Verification items for the finished model (mm, model axes). Face numbers are marked on the shaded views. A direction names the side the tool comes from. Coordinates: 2 decimals unless noted, no trailing zeros. Write each loop counter-clockwise with the first axis right and the second up, starting at its lowest first coordinate (ties: lowest second). Pieces come first, ordered by that corner, then holes. Notation, with made-up numbers: (-23, -3.5) -> (2, -3.5) arc R21 cw to (2, 3.5) -> close; hole circle Ø10 at (61, 38.5). An arc over 180 degrees is marked (long way). Use a Markdown table: item, result. Add a question column.
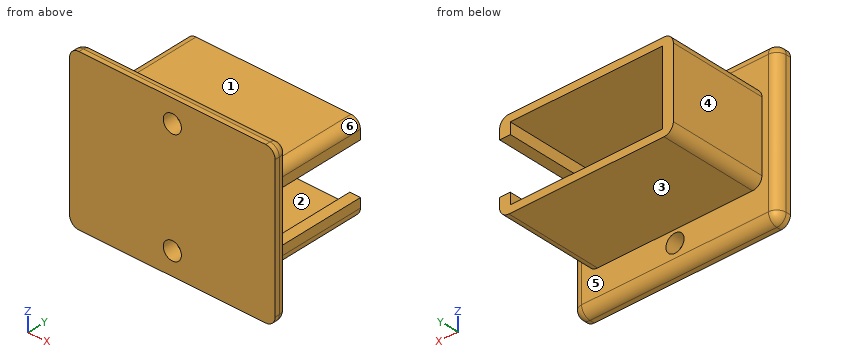
from build123d import *

# Parameters (mm, degrees)
SKETCH1_W           = 55.88
SKETCH1_H           = 43.18
BOSS_EXTRUDE1_DEPTH = 3.81
FILLET1_R           = 2.54
SKETCH3_W           = 47.244
SKETCH3_H           = 24.13
BOSS_EXTRUDE2_DEPTH = 26.67
FILLET2_R           = 2.54
SKETCH6_W           = 41.402
SKETCH6_H           = 20.066
CUT_EXTRUDE1_DEPTH  = 26.67
SKETCH7_R           = 2.461857572
CUT_EXTRUDE2_DEPTH  = 3.81
SKETCH9_W           = 3.778787448
SKETCH9_H           = 13.955771
CUT_EXTRUDE4_DEPTH  = 26.67


with BuildPart() as part:
    # Sketch1 → Boss-Extrude1 (new body)
    with BuildSketch(Plane(origin=(0, 0, 0), x_dir=(1, 0, 0), z_dir=(0, 1, 0))):
        Rectangle(SKETCH1_W, SKETCH1_H)
    extrude(amount=BOSS_EXTRUDE1_DEPTH)

    # Fillet1
    fillet1_edges = [part.edges().sort_by_distance(p)[0] for p in [
        (-27.94, 3.81, 0),
        (0, 3.81, 21.59),
        (27.94, 3.81, 0),
        (27.94, 1.905, 21.59),
        (-27.94, 1.905, 21.59),
        (-27.94, 1.905, -21.59),
        (27.94, 1.905, -21.59),
        (0, 3.81, -21.59),
    ]]
    fillet(fillet1_edges, radius=FILLET1_R)

    # Sketch3 → Boss-Extrude2 (add)
    with BuildSketch(Plane(origin=(0, 3.81, 0), x_dir=(1, 0, 0), z_dir=(0, 1, 0))):
        Rectangle(SKETCH3_W, SKETCH3_H)
    extrude(amount=BOSS_EXTRUDE2_DEPTH)

    # Fillet2
    fillet2_edges = [part.edges().sort_by_distance(p)[0] for p in [
        (23.622, 17.145, 12.065),
        (23.622, 17.145, -12.065),
        (-23.622, 17.145, -12.065),
        (-23.622, 17.145, 12.065),
    ]]
    fillet(fillet2_edges, radius=FILLET2_R)

    # Sketch6 → Cut-Extrude1 (cut)
    with BuildSketch(Plane(origin=(0, 30.48, 0), x_dir=(1, 0, 0), z_dir=(0, 1, 0))):
        Rectangle(SKETCH6_W, SKETCH6_H)
    extrude(amount=-CUT_EXTRUDE1_DEPTH, mode=Mode.SUBTRACT)

    # Sketch7 → Cut-Extrude2 (cut)
    with BuildSketch(Plane(origin=(0, 3.81, 0), x_dir=(1, 0, 0), z_dir=(0, 1, 0))):
        with Locations((0, 15.373463193)):
            Circle(SKETCH7_R)
        with Locations((0, -15.373463193)):
            Circle(SKETCH7_R)
    extrude(amount=-CUT_EXTRUDE2_DEPTH, mode=Mode.SUBTRACT)

    # Sketch9 → Cut-Extrude4 (cut)
    with BuildSketch(Plane(origin=(0, 30.48, 0), x_dir=(1, 0, 0), z_dir=(0, 1, 0))):
        with Locations((21.732606276, 0)):
            Rectangle(SKETCH9_W, SKETCH9_H)
    extrude(amount=-CUT_EXTRUDE4_DEPTH, mode=Mode.SUBTRACT)


solid = part.part
1) Cross-section at D-D on y = 25.5. Record the boundary of the cut face in (x, z) (3 decimals).
2) Cross-section at B-B on y = 2.5. Record the boundary of the cut face in (x, z), then the cut area to 3 significant figures.
3) Cross-section at A-A on x = 0. Record the boundary of the cut face in (y, z) (3 decimals).
4) Cross-section at C-C on z = -1. Record the boundary of the cut face in (x, y), then the cut area to 3 significant figures.
5) Gauge pin test, flat ends, axial feed: pin 1 (11.5 mm diameter, centred on x = -8, z = 0, fed in from +Y); pin 2 (4 mm diameter, centred on y = 25, z = -12, fed in from -X); pin 3 (4.5 mm diameter, centred on x = 0, z = -15.37, fed in from -Y); pin 4 (3 mm diameter, centred on x = 22, y = 10.5, fed in from +Z) (3 decimals). Record the tip position at first contact, or that the pin passes through.
6) Set-up check for the marked faces 1, 2 and 3: record each of +Z, -Z, +X, -X, +Y, -Y from which the full face is reachable in a straight line by a thin tool's end or side.
7) Release check for a two-part mould opening along Z. For the marked faces 4, 5 and 6 record: released by +Z, released by -Z, zero draft, split by the parting line, or undercut.
8) Thickness scan on L1, parallel to Z at x = 0, y = 1; L2, parallel to Z at x = 16.5, y = 12.5 (3 decimals); L3, parallel to X at y = 5, z = 9. Record the ranges inside material, lowest first.
Returned:
| question | item | result |
|---|---|---|
| 1 | outline | (-23.622, -9.525) arc R2.54 ccw to (-21.082, -12.065) -> (21.082, -12.065) arc R2.54 ccw to (23.622, -9.525) -> (23.622, -6.978) -> (20.701, -6.978) -> (20.701, -10.033) -> (-20.701, -10.033) -> (-20.701, 10.033) -> (20.701, 10.033) -> (20.701, 6.978) -> (23.622, 6.978) -> (23.622, 9.525) arc R2.54 ccw to (21.082, 12.065) -> (-21.082, 12.065) arc R2.54 ccw to (-23.622, 9.525) -> close |
| 2 | outline | (-27.62, -19.05) arc R2.22 ccw to (-25.4, -21.27) -> (25.4, -21.27) arc R2.22 ccw to (27.62, -19.05) -> (27.62, 19.05) arc R2.22 ccw to (25.4, 21.27) -> (-25.4, 21.27) arc R2.22 ccw to (-27.62, 19.05) -> close; hole circle Ø4.92 at (0, -15.37); hole circle Ø4.92 at (0, 15.37) |
| 2 | area | 2,310 mm² |
| 3 | outline | (0, -21.59) -> (1.27, -21.59) arc R2.54 ccw to (3.81, -19.05) -> (3.81, -17.835) -> (0, -17.835) -> close; (0, -12.912) -> (3.81, -12.912) -> (3.81, -12.065) -> (30.48, -12.065) -> (30.48, -10.033) -> (3.81, -10.033) -> (3.81, 10.033) -> (30.48, 10.033) -> (30.48, 12.065) -> (3.81, 12.065) -> (3.81, 12.912) -> (0, 12.912) -> close; (0, 17.835) -> (3.81, 17.835) -> (3.81, 19.05) arc R2.54 ccw to (1.27, 21.59) -> (0, 21.59) -> close |
| 4 | outline | (-27.94, 0) -> (27.94, 0) -> (27.94, 1.27) arc R2.54 ccw to (25.4, 3.81) -> (-20.7, 3.81) -> (-20.7, 30.48) -> (-23.62, 30.48) -> (-23.62, 3.81) -> (-25.4, 3.81) arc R2.54 ccw to (-27.94, 1.27) -> close |
| 4 | area | 288 mm² |
| 5 | pin 1 | stops at y = 3.81 |
| 5 | pin 2 | stops at x = -23.58 |
| 5 | pin 3 | passes through |
| 5 | pin 4 | stops at z = 12.065 |
| 6 | face 1 | +Z, +X, -X, +Y |
| 6 | face 2 | +Y |
| 6 | face 3 | -Z, +X, -X, +Y |
| 7 | face 4 | zero draft |
| 7 | face 5 | undercut |
| 7 | face 6 | released by +Z |
| 8 | L1 | z = -21.59 to -17.84, -12.91 to 12.91, 17.84 to 21.59 |
| 8 | L2 | z = -12.065 to -10.033, 10.033 to 12.065 |
| 8 | L3 | x = -23.62 to -20.7, 20.7 to 23.62 |
